Autodesk Inventor part; units mm, degrees
ref_plane "Work Plane1" through (1.525, 0, 0) normal (0, 0, 1) x (1, 0, 0)
ref_plane "YZ Plane" through (0, 0, 0) normal (1, 0, 0) x (0, 1, 0)
ref_plane "XZ Plane" through (0, 0, 0) normal (0, 1, 0) x (-1, 0, 0)
sketch "Sketch1" plane through (0, 0, 0) normal (0, 0, 1) x (1, 0, 0)
  line L0 (0, 11.245) -> (0, 8)
  line L1 (4.5, 8) -> (40, 8)
  line L2 (40, 8) -> (40, 0)
  line L3 (40, 0) -> (-0.8001, 0)
  line L4 (-8.9601, 0) -> (48.16, 0)
  line L5 (-0.8001, 0) -> (-0.8001, 11.245)
  line L6 (-0.8001, 11.245) -> (0, 11.245)
  line L7 (4.5, 8) -> (3.5797, 8)
  line L8 (3.5797, 8) -> (0, 8)
  line L9 (0, -2.249) -> (0, 13.494)
  dimension "d0" = 40
  dimension "d1" = 35.5
  dimension "d2" = 16
  dimension "d9" = 0.8001
  dimension "d10" = 22.49
  dimension "d13" = 0.9203
  dimension "d14" = 16
revolve "Body" add sketch "Sketch1" angle 360 about axis through (40, 0, 0) along (-1, 0, 0)
sketch "Sketch2" plane through (-0.8001, 0, 0) normal (-1, 0, 0) x (0, 0, 1)
  line L0 (0, 13.8564) -> (12, 6.9282)
  line L1 (12, 6.9282) -> (12, -6.9282)
  line L2 (12, -6.9282) -> (0, -13.8564)
  line L3 (0, -13.8564) -> (-12, -6.9282)
  line L4 (-12, -6.9282) -> (-12, 6.9282)
  line L5 (-12, 6.9282) -> (0, 13.8564)
  point P0 (0, 0)
  point P1 (0, 0)
  dimension "d11" = 24
extrude "Head" add sketch "Sketch2" along normal blind 9.2
sketch "Sketch4" plane through (0, 0, 0) normal (0, 0, 1) x (1, 0, 0)
  line L0 (-10.0001, 12) -> (-10.0001, 13.8564)
  line L1 (-10.0001, 13.8564) -> (-8.9283, 13.8564)
  line L2 (-8.9283, 13.8564) -> (-10.0001, 12)
  line L3 (-11.8401, 0) -> (1.0399, 0)
  line L4 (-0.8001, 13.8564) -> (-10.0001, 13.8564)
  line L5 (-10.0001, 6.9282) -> (-10.0001, 13.8564)
  dimension "d5" = 30
  dimension "d19" = 24
revolve "Chamfer1" cut sketch "Sketch4" angle 360 about axis through (-10, 0, 0) along (1, 0, 0)
thread "Thread"
chamfer "Chamfer2" distance 0.9202 distance2 0.9203 1 edges at (40, -8, 0) measured on face at (40, -0.1598, 1.3157)
ref_plane "Work Plane1" through (1.525, 0, 0) normal (0, 0, 1) x (1, 0, 0)
equation "\"d11\" = SW"
equation "\"d3\" = KOH - SD"
equation "\"d15\" = GEL"
equation "\"d6\" = -0.5 * SPD + 0.5 * GD"
equation "\"d0\" = NLG"
equation "\"d1\" = GEL"
equation "\"d2\" = GD"
equation "\"d10\" = SD2"
equation "\"d14\" = BDM"
equation "\"d5\" = ANG1"
equation "\"d19\" = SW0"
equation "\"NLG\" = 40"
equation "\"GD\" = NND"
equation "\"BDM\" = NND"
equation "\"KOH\" = 10"
equation "\"GEL\" = 35.5"
equation "\"SW\" = 24"
equation "\"SW0\" = 24"
equation "\"SPD\" = NND - 1.2269 * PTC"
equation "\"SD2\" = 22.49"
equation "\"SD\" = 0.8"
equation "\"ANG1\" = 30deg"
equation "\"GAL\" = 0.61345 * PTC"
equation "\"GUL\" = 0.61345 * PTC"
equation "\"RR\" = 0.6"
equation "\"GD1\" = THREADDIA - 1.2269 * PTC"
equation "\"THREADDIA\" = 16"
equation "\"SDH\" = SD2"
equation "\"TOA\" = 30deg"
equation "\"PTC\" = 1.5"
equation "\"NND\" = 16"
equation "\"E0\" = 1.155 * SW"
properties part number "ISO 8676 - M16 x 1,5 x 40" material "Stainless Steel, 440C"
Work out the finished part from the listing and answer in its coordinate system (mm). A direction names the side the tool comes from. Give positions to 0.01 mm unless a question says otherwise; leave off trailing zeros. Loops run counter-clockwise (first coordinate to the right, second up) from the corner with the lowest first, then second, coordinate; pieces in that order, holes last. Notation, with made-up numbers: (67.25, 80) -> (103.25, 80) arc R12 cw to (103.25, 89) -> close; hole circle Ø9 at (65.5, -34.75). An arc over 180 degrees is marked (long way). Put each result on its own line as item: value. Start each with the question number.
Item 1: The part is cut by section A-A (x = 23.5). Give the vertices of the cut face in (y, z), then the cut area to 3 significant figures.
Item 2: Each of these flat-tipped pins is pushed along its axis until it touches: P1, Ø10, axis at x = 24.5, z = 5, coming from the -Y side; P2, Ø3, axis at x = 31, y = 7, coming from the -Z side; P3, Ø4, axis at x = 25, z = -2, coming from the +Y side. Where does it stop, or does it pass through?
Item 3: Which of the six approach directions +Z, -Z, +X, -X, +Y, -Y give full straight-line access (tool end or side, diameter ignored) to faces 1 (the face through (-5.336, 10.344, -6.084)), 2 (the face through (-0.8, 11.4, -0.1))?
Item 4: Find the intervals of material crossed by L1, parallel to X at y = -2.5, z = 8; L2, parallel to X at y = 11.5, z = 2.5; L3, parallel to Z at x = -5, y = 10.25, in increasing order. Write a range as [from, to].
Answers below:
1. outline: circle Ø16 at (0, 0)
1. area: 201 mm2
2. P1: y = -8
2. P2: z = -5.81
2. P3: y = 8
3. face 1: -Z, +X, -X, +Y
3. face 2: +X
4. L1: [-10, 0]
4. L2: [-10, -0.8]
4. L3: [-6.25, 6.25]
